Model file for the job. Use its own axes, mm. A direction names the side the tool comes from. Coordinates: 2 decimals unless noted, no trailing zeros. Write each loop counter-clockwise with the first axis right and the second up, starting at its lowest first coordinate (ties: lowest second). Pieces come first, ordered by that corner, then holes. Notation, with made-up numbers: (69.25, 81) - (77.25, 81) arc R33 ccw to (77.25, 110) - close; hole circle Ø8 at (82.25, -37.5). An arc over 180 degrees is marked (long way). Put each result on its own line as item: value. Start each with the question number.
1. Drop flat-ended pins along their axis: P1, Ø3.5, axis at x = -4.6, z = 40.04, coming from the -Y side; P2, Ø1, axis at x = -5, y = -2, coming from the -Z side; P3, Ø4, axis at x = -20, z = 52.5, coming from the +Y side. Give the stop position or say it passes through.
2. Saw through at B-B, the plane z = 10. Write the cut outline in (x, y), plus the area to 4 significant figures.
3. Saw through at C-C, the plane y = 3.25. Write the cut outline in (x, z).
4. Saw through at D-D, the plane x = -15.5. Write the cut outline in (y, z), plus the area to 3 significant figures.
5. Pull direction Z, two halves, no side cores. Call faces 1 (the face through (0, 0, 34)), 2 (the face through (-28.869, 3.521, 43.214)), 3 (the face through (-13, -4, 50)): released by +Z, released by -Z, zero draft, split by the parting line, or undercut.
6. Saw through at A-A, the plane x = -8.6. Write the cut outline in (y, z).
7. Drill centre lines: L1, parallel to X at y = 0.75, z = 52.5; L2, parallel to Y at x = -25.75, z = 53; L3, parallel to Z at x = -9.5, y = 3.25. Where is each one in solid material? Low to high. Write a range as from..to.
8. Which spindle directions (+Z, -Z, +X, -X, +Y, -Y) get a long thin tool onto all of the face, cutting with end or side? Do faces 4 (the face through (-21.996, 3.521, 25.538)), 5 (the face through (-5, -5.4, 40)), 6 (the face through (-13, -4, 29.5)), 7 (the face through (-25, -4, 40)). Say none if no direction does.
```python
from build123d import *

# Parameters (mm, degrees)
SKETCH_1_W          = 30
SKETCH_1_H          = 55
EXTRUDE_1_DEPTH     = 5
SKETCH_4_R          = 1.5
CUT_EXTRUDE_1_DEPTH = 63.84902545
SKETCH_4_3_R        = 2.25
CUT_EXTRUDE_2_DEPTH = 3
SKETCH_5_W          = 25
SKETCH_5_H          = 20.5
EXTRUDE_2_DEPTH     = 8
SKETCH_6_R          = 3.1
CUT_EXTRUDE_3_DEPTH = 2.6
SKETCH_6_3_R        = 1.1
CUT_EXTRUDE_4_DEPTH = 64.984373092


with BuildPart() as part:
    # 草图1 → 凸台-拉伸1 (new body)
    with BuildSketch(Plane(origin=(0, 0, 0), x_dir=(1, 0, 0), z_dir=(0, 1, 0))):
        with Locations((-15, -27.5)):
            Rectangle(SKETCH_1_W, SKETCH_1_H)
    extrude(amount=EXTRUDE_1_DEPTH)

    # 草图4 → 切除-拉伸1 (cut, through all)
    with BuildSketch(Plane(origin=(0, 5, 0), x_dir=(1, 0, 0), z_dir=(0, 1, 0))):
        with Locations(Location((-27.5, -10, 0), (0, 0, 270))):
            Circle(SKETCH_4_R)
        with Locations(Location((-27.5, -45, 0), (0, 0, 270))):
            Circle(SKETCH_4_R)
        with Locations(Location((-20, -52.5, 0), (0, 0, 270))):
            Circle(SKETCH_4_R)
        with Locations(Location((-8.6, -52.5, 0), (0, 0, 270))):
            Circle(SKETCH_4_R)
        with Locations(Location((-8.6, -24.5, 0), (0, 0, 270))):
            Circle(SKETCH_4_R)
        with Locations(Location((-20, -24.5, 0), (0, 0, 270))):
            Circle(SKETCH_4_R)
    extrude(amount=-CUT_EXTRUDE_1_DEPTH, mode=Mode.SUBTRACT)

    # 草图4<3> → 切除-拉伸2 (cut)
    with BuildSketch(Plane(origin=(0, 5, 0), x_dir=(1, 0, 0), z_dir=(0, 1, 0))):
        with Locations(Location((-27.5, -10, 0), (0, 0, 270))):
            Circle(SKETCH_4_3_R)
        with Locations(Location((-27.5, -45, 0), (0, 0, 270))):
            Circle(SKETCH_4_3_R)
        with Locations(Location((-20, -52.5, 0), (0, 0, 270))):
            Circle(SKETCH_4_3_R)
        with Locations(Location((-8.6, -52.5, 0), (0, 0, 270))):
            Circle(SKETCH_4_3_R)
        with Locations(Location((-8.6, -24.5, 0), (0, 0, 270))):
            Circle(SKETCH_4_3_R)
        with Locations(Location((-20, -24.5, 0), (0, 0, 270))):
            Circle(SKETCH_4_3_R)
    extrude(amount=-CUT_EXTRUDE_2_DEPTH, mode=Mode.SUBTRACT)

    # 草图5 → 凸台-拉伸2 (add)
    with BuildSketch(Plane.XZ):
        with Locations((-12.5, 39.75)):
            Rectangle(SKETCH_5_W, SKETCH_5_H)
    extrude(amount=EXTRUDE_2_DEPTH)

    # 草图6 → 切除-拉伸3 (cut)
    with BuildSketch(Plane.XZ.offset(8)):
        with Locations(Location((-4.6, 40.035904331, 0), (0, 0, 270))):
            Circle(SKETCH_6_R)
    extrude(amount=-CUT_EXTRUDE_3_DEPTH, mode=Mode.SUBTRACT)

    # 草图6<3> → 切除-拉伸4 (cut, through all)
    with BuildSketch(Plane.XZ.offset(8)):
        with Locations(Location((-15.5, 43.701964887, 0), (0, 0, 270))):
            Circle(SKETCH_6_3_R)
    extrude(amount=-CUT_EXTRUDE_4_DEPTH, mode=Mode.SUBTRACT)


solid = part.part
```
Final values:
1. P1: stops at y = -5.4
1. P2: stops at z = 29.5
1. P3: stops at y = 2
2. outline: (-30, 0) - (-29, 0) - (-29, 2) - (-29.75, 2) - (-29.75, 5) - (-30, 5) - close; (-26, 0) - (0, 0) - (0, 5) - (-25.25, 5) - (-25.25, 2) - (-26, 2) - close
2. area: 130.5 mm²
3. outline: (-30, 0) - (0, 0) - (0, 55) - (-30, 55) - close; hole circle Ø4.5 at (-27.5, 10); hole circle Ø4.5 at (-27.5, 45); hole circle Ø4.5 at (-20, 24.5); hole circle Ø4.5 at (-20, 52.5); hole circle Ø2.2 at (-15.5, 43.7); hole circle Ø4.5 at (-8.6, 24.5); hole circle Ø4.5 at (-8.6, 52.5)
4. outline: (-8, 29.5) - (0, 29.5) - (0, 0) - (5, 0) - (5, 42.6) - (-8, 42.6) - close; (-8, 44.8) - (5, 44.8) - (5, 55) - (0, 55) - (0, 50) - (-8, 50) - close
4. area: 410 mm²
5. face 1: zero draft
5. face 2: undercut
5. face 3: released by +Z
6. outline: (-8, 29.5) - (0, 29.5) - (0, 26) - (2, 26) - (2, 26.75) - (5, 26.75) - (5, 50.25) - (2, 50.25) - (2, 51) - (0, 51) - (0, 50) - (-8, 50) - close; (0, 0) - (5, 0) - (5, 22.25) - (2, 22.25) - (2, 23) - (0, 23) - close; (0, 54) - (2, 54) - (2, 54.75) - (5, 54.75) - (5, 55) - (0, 55) - close
7. L1: x = -30..-21.5, -18.5..-10.1, -7.1..0
7. L2: y = 0..5
7. L3: z = 0..22.44, 26.56..50.44, 54.56..55
8. face 4: +Y
8. face 5: -Y
8. face 6: -Z, +X, -X, -Y
8. face 7: +Z, -Z, -X, -Y
